from build123d import *

# Parameters (mm, degrees)
SKETCH1_W           = 44
SKETCH1_H           = 44
BOSS_EXTRUDE1_DEPTH = 16
SKETCH3_W           = 40
SKETCH3_H           = 40
CUT_EXTRUDE1_DEPTH  = 13
SKETCH5_W           = 23
SKETCH5_H           = 11
CUT_EXTRUDE2_DEPTH  = 13
SKETCH6_W           = 16
SKETCH6_H           = 6
CUT_EXTRUDE3_DEPTH  = 10
SKETCH7_W           = 10
SKETCH7_H           = 12
CUT_EXTRUDE4_DEPTH  = 5
SKETCH8_W           = 4.5
SKETCH8_H           = 3
SKETCH8_W_2         = 9
BOSS_EXTRUDE2_DEPTH = 10
SKETCH9_R           = 1
CUT_EXTRUDE5_DEPTH  = 10
SKETCH10_W          = 9
SKETCH10_H          = 3
SKETCH10_W_2        = 4.5
BOSS_EXTRUDE3_DEPTH = 10
SKETCH11_R          = 1
CUT_EXTRUDE6_DEPTH  = 10


with BuildPart() as part:
    # Sketch1 → Boss-Extrude1 (new body)
    with BuildSketch(Plane.XY):
        with Locations((22, 22)):
            Rectangle(SKETCH1_W, SKETCH1_H)
    extrude(amount=BOSS_EXTRUDE1_DEPTH)

    # Sketch3 → Cut-Extrude1 (cut)
    with BuildSketch(Plane(origin=(0, 0, 0), x_dir=(-1, 0, 0), z_dir=(0, 0, -1))):
        with Locations((-22.063776274, 22)):
            Rectangle(SKETCH3_W, SKETCH3_H)
    extrude(amount=-CUT_EXTRUDE1_DEPTH, mode=Mode.SUBTRACT)

    # Sketch5 → Cut-Extrude2 (cut)
    with BuildSketch(Plane.XY.offset(16)):
        with Locations((18.5, 38.5)):
            Rectangle(SKETCH5_W, SKETCH5_H)
    extrude(amount=-CUT_EXTRUDE2_DEPTH, mode=Mode.SUBTRACT)

    # Sketch6 → Cut-Extrude3 (cut)
    with BuildSketch(Plane.XY.offset(16)):
        with Locations((22, 3)):
            Rectangle(SKETCH6_W, SKETCH6_H)
    extrude(amount=-CUT_EXTRUDE3_DEPTH, mode=Mode.SUBTRACT)

    # Sketch7 → Cut-Extrude4 (cut)
    with BuildSketch(Plane(origin=(44, 0, 0), x_dir=(0, 0, -1), z_dir=(1, 0, 0))):
        with Locations((-5, 22)):
            Rectangle(SKETCH7_W, SKETCH7_H)
    extrude(amount=-CUT_EXTRUDE4_DEPTH, mode=Mode.SUBTRACT)

    # Sketch8 → Boss-Extrude2 (add)
    with BuildSketch(Plane(origin=(0, 0, 0), x_dir=(-1, 0, 0), z_dir=(0, -1, 0))):
        with Locations((-6.75, -1.5)):
            Rectangle(SKETCH8_W, SKETCH8_H)
        with Locations((-37.5, -1.5)):
            Rectangle(SKETCH8_W_2, SKETCH8_H)
    extrude(amount=BOSS_EXTRUDE2_DEPTH)

    # Sketch9 → Cut-Extrude5 (cut)
    with BuildSketch(Plane.XY.offset(3)):
        with Locations((6.5, -6.077320914)):
            Circle(SKETCH9_R)
        with Locations((37.5, -6.077320914)):
            Circle(SKETCH9_R)
    extrude(amount=-CUT_EXTRUDE5_DEPTH, mode=Mode.SUBTRACT)

    # Sketch10 → Boss-Extrude3 (add)
    with BuildSketch(Plane(origin=(0, 44, 0), x_dir=(1, 0, 0), z_dir=(0, 1, 0))):
        with Locations((37.5, -1.5)):
            Rectangle(SKETCH10_W, SKETCH10_H)
        with Locations((6.75, -1.5)):
            Rectangle(SKETCH10_W_2, SKETCH10_H)
    extrude(amount=BOSS_EXTRUDE3_DEPTH)

    # Sketch11 → Cut-Extrude6 (cut)
    with BuildSketch(Plane.XY.offset(3)):
        with Locations((37.5, 49.031327524)):
            Circle(SKETCH11_R)
        with Locations((6.5, 49.031327524)):
            Circle(SKETCH11_R)
    extrude(amount=-CUT_EXTRUDE6_DEPTH, mode=Mode.SUBTRACT)


solid = part.part
Can you work these out from the model? Positions are in its coordinate system, mm. A direction names the side the tool comes from. Give positions to 0.01 mm unless a question says otherwise; leave off trailing zeros. Order: outer loops, then holes, each group sorted by start corner. A loop starts at its lowest first (then second) coordinate and runs counter-clockwise, first axis right, second up. Notation, with made-up numbers: M 8,-34.75 L 17,-34.75 A17 cw 17,-11.75 Z; hole C 76.5,-20 d7. An arc over 180 degrees is marked long. One line per item, written item: value.
Item 1: If we mould it in two halves opening along Y, with no side actions, what happens to faces 1 (the face through (2.064, 22, 6)), 2 (the face through (18, 33, 15)), 3 (the face through (24, 43, 0))? For each: pulls with the +Y half, pulls with the -Y half, needs draft (parallel to the pull), parting line crosses it, or undercut.
Verdict:
face 1: undercut
face 2: pulls with the +Y half
face 3: needs draft
Item 2: For faces 4 (the face through (38, -5, 3)), 5 (the face through (27, 42, 2)), 6 (the face through (22, 6, 15)), 7 (the face through (43, 28, 5)), 8 (the face through (7, 41, 14)), which set-ups out of +Z, -Z, +X, -X, +Y, -Y let a thin tool reach every point of the face, with its end or its side?
Verdict:
face 4: +Z, +X, -X, -Y
face 5: -Z
face 6: +Z, -Z, -Y
face 7: -Z, +X
face 8: +Z, +Y
Item 3: Please list where these lines run through material, in increasing order: line 1 (Y direction, x = 37.5, z = 1); line 2 (X direction, y = 30.5, z = 9.75); line 3 (Y direction, x = 42.5, z = 2.5).
Verdict:
line 1: -10 to -7.08, -5.08 to 2, 42 to 48.03, 50.03 to 54
line 2: 0 to 2.06, 42.06 to 44
line 3: 0 to 16, 28 to 44
Item 4: If we section it at A-A on x = 26.5: Write out the boundary of the cut face in (y, z), and give its area (3 significant figures).
Verdict:
outline: M 0,0 L 2,0 L 2,6 L 0,6 Z; M 6,13 L 33,13 L 33,16 L 6,16 Z; M 42,0 L 44,0 L 44,3 L 42,3 Z
area: 99.0 mm2
Item 5: If we section it at C-C on z = 12: Write out the boundary of the cut face in (x, y), and give its area (3 significant figures).
Verdict:
outline: M 0,0 L 14,0 L 14,2 L 2.06,2 L 2.06,42 L 7,42 L 7,44 L 0,44 Z; M 30,0 L 44,0 L 44,44 L 30,44 L 30,42 L 42.06,42 L 42.06,2 L 30,2 Z
area: 258 mm2
Item 6: For pin 1 (1 mm diameter, centred on x = 43, z = 3, fed in from -Y); pin 2 (0.9 mm diameter, centred on y = 49, z = 2, fed in from -X); pin 3 (0.9 mm diameter, centred on y = -6, z = 2, fed in from +X); pin 4 (1.2 mm diameter, centred on x = 37.5, y = -6.08, fed in from -Z), each with a flat end and sliding along its axis, tell me the tip position at first contact or that it passes through.
Verdict:
pin 1: y = 0
pin 2: x = 4.5
pin 3: x = 42
pin 4: through
Item 7: If we section it at D-D on y = 26: Write out the boundary of the cut face in (x, z).
Verdict:
outline: M 0,0 L 2.06,0 L 2.06,13 L 42.06,13 L 42.06,10 L 44,10 L 44,16 L 0,16 Z
Item 8: If we section it at B-B on y = 37: Write out the boundary of the cut face in (x, z), and give its area (3 significant figures).
Verdict:
outline: M 0,0 L 2.06,0 L 2.06,13 L 7,13 L 7,16 L 0,16 Z; M 30,13 L 42.06,13 L 42.06,0 L 44,0 L 44,16 L 30,16 Z
area: 115 mm2
